from build123d import *

# Parameters (mm, degrees)
BOSS_EXTRUDE1_DEPTH       = 8
CUT_EXTRUDE1_DEPTH        = 8
SKETCH7_R                 = 1.5
CUT_EXTRUDE4_DEPTH        = 2
SKETCH9_R                 = 2.5
CUT_EXTRUDE5_DEPTH        = 15
CUT_EXTRUDE2_DEPTH        = 21
CUT_EXTRUDE3_DEPTH        = 21
M2X0_4_TAPPED_HOLE1_D     = 1.6
M2X0_4_TAPPED_HOLE1_DEPTH = 8
M2X0_4_TAPPED_HOLE1_TIP   = 0.480688495


with BuildPart() as part:
    # Sketch1 → Boss-Extrude1 (new body)
    with BuildSketch(Plane.XY):
        Polygon((0, 0), (0, 42), (20, 42), (20, 16), (40, 16), (40, 8), align=None)
    extrude(amount=BOSS_EXTRUDE1_DEPTH)

    # Sketch2 → Cut-Extrude1 (cut)
    with BuildSketch(Plane.XY.offset(8)):
        Polygon((15, 42), (15, 35), (0, 28), (0, 42), align=None)
    extrude(amount=-CUT_EXTRUDE1_DEPTH, mode=Mode.SUBTRACT)

    # Sketch7 → Cut-Extrude4 (cut)
    with BuildSketch(Plane(origin=(0, 16, 0), x_dir=(1, 0, 0), z_dir=(0, 1, 0))):
        with Locations((34, -4)):
            Circle(SKETCH7_R)
        with Locations((26, -4)):
            Circle(SKETCH7_R)
    extrude(amount=-CUT_EXTRUDE4_DEPTH, mode=Mode.SUBTRACT)

    # Sketch9 → Cut-Extrude5 (cut, through all)
    with BuildSketch(Plane(origin=(0, 14, 0), x_dir=(1, 0, 0), z_dir=(0, 1, 0))):
        with Locations((34, -4)):
            Circle(SKETCH9_R)
        with Locations((26, -4)):
            Circle(SKETCH9_R)
    extrude(amount=-CUT_EXTRUDE5_DEPTH, mode=Mode.SUBTRACT)

    # Sketch5 → Cut-Extrude2 (cut, through all)
    with BuildSketch(Plane(origin=(20, 0, 0), x_dir=(0, 0, -1), z_dir=(1, 0, 0))):
        Polygon((-8, 42), (-4, 42), (-8, 38), align=None)
    extrude(amount=-CUT_EXTRUDE2_DEPTH, mode=Mode.SUBTRACT)

    # Sketch6 → Cut-Extrude3 (cut, through all)
    with BuildSketch(Plane(origin=(20, 0, 0), x_dir=(0, 0, -1), z_dir=(1, 0, 0))):
        Polygon((0, 42), (-4, 42), (0, 38), align=None)
    extrude(amount=-CUT_EXTRUDE3_DEPTH, mode=Mode.SUBTRACT)

    # M2x0.4 Tapped Hole1
    with Locations(Plane(origin=(0, 24, 4), x_dir=(0, 0, -1), z_dir=(-1, 0, 0))):
        with Locations((0, 0), (0, 8), (0, 16)):
            Hole(M2X0_4_TAPPED_HOLE1_D / 2, depth=M2X0_4_TAPPED_HOLE1_DEPTH)
            with Locations((0, 0, -(M2X0_4_TAPPED_HOLE1_DEPTH + M2X0_4_TAPPED_HOLE1_TIP / 2))):  # 118° drill point
                Cone(0, M2X0_4_TAPPED_HOLE1_D / 2, M2X0_4_TAPPED_HOLE1_TIP, mode=Mode.SUBTRACT)


solid = part.part
Can you work these out from the model? Positions are in its coordinate system, mm. A direction names the side the tool comes from. Give positions to 0.01 mm unless a question says otherwise; leave off trailing zeros. Loops run counter-clockwise (first coordinate to the right, second up) from the corner with the lowest first, then second, coordinate; pieces in that order, holes last. Notation, with made-up numbers: (23, 68) -> (52, 68) arc R23 cw to (52, 88) -> close; hole circle Ø1 at (75.5, 32). An arc over 180 degrees is marked (long way). Return JSON: item names as keys, results as strings.
Q1. For pin 1 Ø2.5 at (x, z) = (27, 4.5) entering from -Y; pin 2 Ø1 at (y, z) = (8, 4) entering from -X; pin 3 Ø1.5 at (x, z) = (28, 4) entering from +Y, each with a flat end and sliding along its axis, tell me the tip position at first contact or that it passes through.
Checks:
{"pin 1": "stops at y = 14", "pin 2": "stops at x = 8.18", "pin 3": "stops at y = 16"}
Q2. We'd pull the mould along Z, two halves only. Please class faces 1 (the face through (30, 16, 4)), 2 (the face through (23.5, 9.4, 3.9)), 3 (the face through (16, 15, 8)), 4 (the face through (16, 15, 0)): released by +Z, released by -Z, zero draft, split by the parting line, or undercut.
Checks:
{"face 1": "zero draft", "face 2": "undercut", "face 3": "released by +Z", "face 4": "released by -Z"}
Q3. I want a section at B-B, the plane x = 34. List the corners of the cut face in (y, z) for me, then the cut area to 3 significant figures.
Checks:
{"outline": "(6.8, 0) -> (16, 0) -> (16, 2.5) -> (14, 2.5) -> (14, 1.5) -> (6.8, 1.5) -> close; (6.8, 6.5) -> (14, 6.5) -> (14, 5.5) -> (16, 5.5) -> (16, 8) -> (6.8, 8) -> close", "area": "31.6 mm2"}
Q4. I need wall thicknesses on probe 1 along Z at (x, y) = (26, 9); probe 2 along Z at (x, y) = (26, 15.5); probe 3 along X at (y, z) = (10, 3). Which ranges of each line are inside material? Lowest first, please.
Checks:
{"probe 1": "z = 0 to 1.5, 6.5 to 8", "probe 2": "z = 0 to 2.5, 5.5 to 8", "probe 3": "x = 0 to 23.71, 28.29 to 31.71, 36.29 to 40"}
Q5. On a 3-axis mill with a long thin cutter (end or side, diameter ignored), from which of +Z, -Z, +X, -X, +Y, -Y can I reach the whole of each face in a straight line? I mean faces 5 (the face through (32.8, 15, 4.9)), 6 (the face through (15, 38, 4)), 7 (the face through (36, 14, 4)), 8 (the face through (4.06, 7.46, 3.41)). Say none if no direction works.
Checks:
{"face 5": "+Y, -Y", "face 6": "+Z, -Z, -X, +Y", "face 7": "-Y", "face 8": "-X"}
Q6. I want a section at A-A, the plane y = 9.5. List the corners of the cut face in (x, z) for me.
Checks:
{"outline": "(0, 0) -> (40, 0) -> (40, 8) -> (0, 8) -> close; hole circle Ø5 at (26, 4); hole circle Ø5 at (34, 4)"}
Q7. I want a section at D-D, the plane x = 5. List the corners of the cut face in (y, z) for me, then the cut area to 3 significant figures.
Checks:
{"outline": "(1, 0) -> (30.33, 0) -> (30.33, 8) -> (1, 8) -> close; hole circle Ø1.6 at (8, 4); hole circle Ø1.6 at (16, 4); hole circle Ø1.6 at (24, 4)", "area": "229 mm2"}
Q8. I want a section at C-C, the plane y = 14.5. List the corners of the cut face in (x, z) for me, then the cut area to 3 significant figures.
Checks:
{"outline": "(0, 0) -> (40, 0) -> (40, 8) -> (0, 8) -> close; hole circle Ø3 at (26, 4); hole circle Ø3 at (34, 4)", "area": "306 mm2"}
